For this review, use the dimensioned drawing (mm, ordinates from the lowest corner) and the shaded views. Round coordinates to 2 decimals unless told otherwise and drop trailing zeros. Loops run counter-clockwise (first coordinate to the right, second up) from the corner with the lowest first, then second, coordinate; pieces in that order, holes last. Notation, with made-up numbers: M -39.75,6 L 14.25,6 A12 ccw 14.25,14 Z; hole C 45,67 d3. An arc over 180 degrees is marked long. Answer as a JSON object with one key per item and string values. Group by question number.
Item 1: Consider section A-A (x = 25). Give the boundary of the cut face in (y, z), and give its area (3 significant figures).
Item 2: Consider section C-C (z = 1.95). Give the boundary of the cut face in (x, y), and give its area (3 significant figures).
Item 3: To check wall thickness, follow line 1 (Y direction, x = 25, z = 2.75); line 2 (Y direction, x = 28, z = 1.55); line 3 (X direction, y = 19, z = 1.1). State the ranges of each line that lie inside material, in increasing order.
Item 4: Insertion check: P1, Ø9.5, axis at x = 25, y = 25, coming from the +Z side. The pin has a flat end and moves straight along its axis. Give the tip position at first contact, or say it passes through.
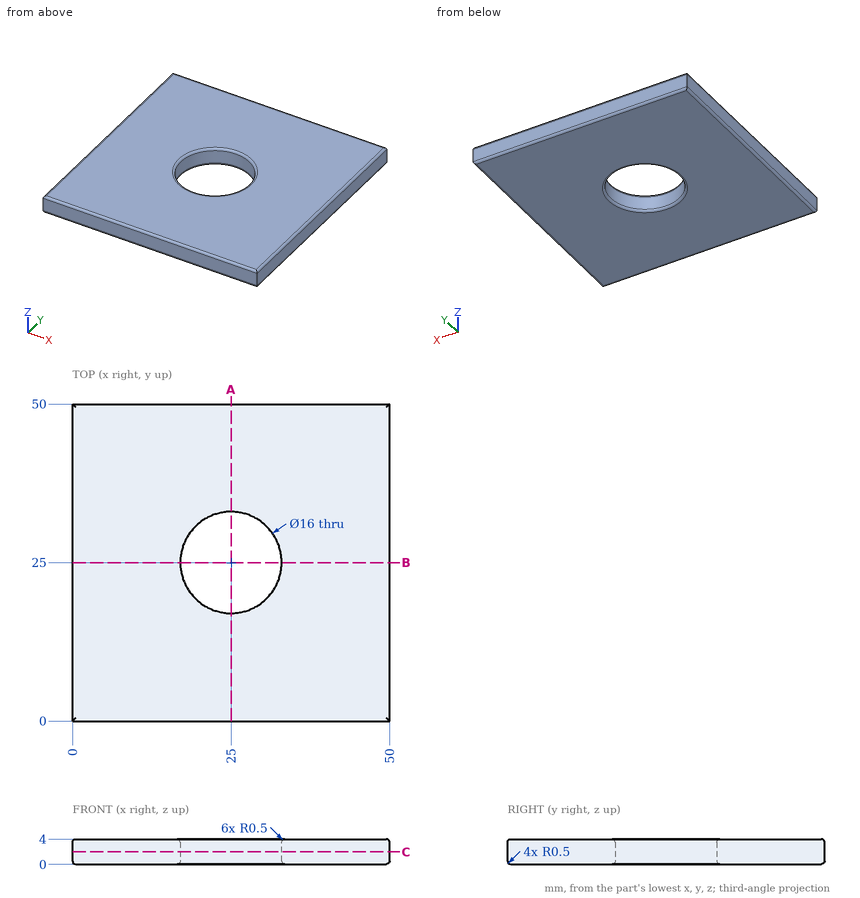
Geometry results:
{
 "1": {"outline": "M 0,0.5 A0.5 ccw 0.5,0 L 16.5,0 A0.5 ccw 17,0.5 L 17,3.5 A0.5 ccw 16.5,4 L 0.5,4 A0.5 ccw 0,3.5 Z; M 33,0.5 A0.5 ccw 33.5,0 L 49.5,0 A0.5 ccw 50,0.5 L 50,3.5 A0.5 ccw 49.5,4 L 33.5,4 A0.5 ccw 33,3.5 Z", "area": "136 mm^2"},
 "2": {"outline": "M 0,0 L 50,0 L 50,50 L 0,50 Z; hole C 25,25 d16", "area": "2,300 mm^2"},
 "3": {"line 1": "y = 0 to 17, 33 to 50", "line 2": "y = 0 to 17.58, 32.42 to 50", "line 3": "x = 0 to 19.71, 30.29 to 50"},
 "4": {"P1": "passes through"}
}
